```python
from build123d import *

# Parameters (mm, degrees)
F0_W        = 35
F0_H        = 20
F1_DEPTH    = 20
F2_W        = 30
F2_H        = 17.5
F3_DEPTH    = 25
F4_R        = 6
F5_DEPTH    = 5
F6_T1_DEPTH = 32.5
F7_R        = 7.5
F7_R_2      = 1.25
F8_DEPTH    = 25
F9_R        = 1.25
F10_DEPTH   = 25
F11_DEPTH   = 5
F13_DEPTH   = 5


# Not quite as in the source:
# - a fillet or chamfer that OpenCascade refuses, or shapes differently, is made with other operations: its cross-section is extruded or revolved along the edge and cut away or added


with BuildPart() as f1:
    # F0 (on Top) → F1 (new body)
    with BuildSketch(Plane.XY):
        with Locations((17.5, 10)):
            Rectangle(F0_W, F0_H)
    extrude(amount=F1_DEPTH)

    # F2 (on face) → F3 (cut)
    with BuildSketch(Plane.XY.offset(20)):
        with Locations((17.5, 11.25)):
            Rectangle(F2_W, F2_H)
    extrude(amount=-F3_DEPTH, mode=Mode.SUBTRACT)

    # F4 (on face) → F5 (cut)
    with BuildSketch(Plane(origin=(0, 0, 0), x_dir=(0, -1, 0), z_dir=(-1, 0, 0))):
        with Locations((-7.5, 10)):
            Circle(F4_R)
        Polygon((-20, 20), (-20, 10), (-10, 20), align=None)
    extrude(amount=-F5_DEPTH, mode=Mode.SUBTRACT)

    # F6: fillet of radius 2.5 on 2 edges, made by hand

    # F6_s2 → F6_t1 (cut)
    with BuildSketch(Plane.XY.offset(-6.25)):
        with BuildLine():
            ThreePointArc((0, 2.5), (0.732233047, 0.732233047), (2.5, 0))
            Line((2.5, 0), (0, 0))
            Line((0, 0), (0, 2.5))
        make_face()
        with BuildLine():
            ThreePointArc((32.5, 0), (34.267766953, 0.732233047), (35, 2.5))
            Line((35, 2.5), (35, 0))
            Line((35, 0), (32.5, 0))
        make_face()
    extrude(amount=F6_T1_DEPTH, mode=Mode.SUBTRACT)

    # F7 (on face) → F8 (cut)
    with BuildSketch(Plane.XZ):
        with Locations((17.5, 10)):
            Circle(F7_R)
        with Locations((28.5, 16)):
            Circle(F7_R_2)
        with Locations((28.5, 10)):
            Circle(F7_R_2)
        with Locations((28.5, 4)):
            Circle(F7_R_2)
    extrude(amount=-F8_DEPTH, mode=Mode.SUBTRACT)

    # F9 (on face) → F10 (cut)
    with BuildSketch(Plane.XZ):
        with Locations((6.5, 4)):
            Circle(F9_R)
        with Locations((6.5, 10)):
            Circle(F9_R)
        with Locations((6.5, 16)):
            Circle(F9_R)
    extrude(amount=-F10_DEPTH, mode=Mode.SUBTRACT)

    # F11 (add): a face of the model
    f11_faces = [f1.faces().sort_by_distance(p)[0] for p in [
        (33.75, 20, 10),
    ]]
    extrude(f11_faces, amount=F11_DEPTH)

    # F12 (on face) → F13 (cut)
    with BuildSketch(Plane.YZ.offset(35)):
        with BuildLine():
            Line((8, 7.5), (20, 7.5))
            ThreePointArc((20, 7.5), (22.5, 10), (20, 12.5))
            Line((20, 12.5), (8, 12.5))
            ThreePointArc((8, 12.5), (5.5, 10), (8, 7.5))
        make_face()
        with BuildLine():
            Line((15.75, 16), (25, 16))
            Line((25, 16), (25, 20))
            Line((25, 20), (13.75, 20))
            Line((13.75, 20), (13.75, 18))
            ThreePointArc((13.75, 18), (14.3357864376, 16.5857864376), (15.75, 16))
        make_face()
        with BuildLine():
            Line((25, 0), (25, 4))
            Line((25, 4), (15.75, 4))
            ThreePointArc((15.75, 4), (14.3357864376, 3.4142135624), (13.75, 2))
            Line((13.75, 2), (13.75, 0))
            Line((13.75, 0), (25, 0))
        make_face()
    extrude(amount=-F13_DEPTH, mode=Mode.SUBTRACT)


solid = f1.part
```
The listing builds one solid part. Answer for the finished solid, in the listing's coordinates (mm). A direction names the side the tool comes from. Coordinates: 2 decimals unless noted, no trailing zeros. Order: outer loops, then holes, each group sorted by start corner. A loop starts at its lowest first (then second) coordinate and runs counter-clockwise, first axis right, second up. Notation, with made-up numbers: M 46,-23 L 57,-23 A19 cw 57,-13 Z; hole C -34.75,-28.75 d4. An arc over 180 degrees is marked long. Answer as a JSON object with one key per item and string values. Group by question number.
1. Straight lines are drawn through the part: line 1 (Z direction, x = 28.5, y = 1.65); line 2 (X direction, y = 6, z = 18.5); line 3 (Z direction, x = 33, y = 10.75). For each, find the intervals that lie inside material, in ascending order.
2. Section D-D on x = 15 is taken. Write down the section's boundary in (y, z), then the cut area to 3 significant figures.
3. Section C-C on z = 12 is taken. Write down the section's boundary in (x, y).
4. Section A-A on y = 17 is taken. Write down the section's boundary in (x, z), then the cut area to 3 significant figures.
5. Section B-B on x = 6.5 is taken. Write down the section's boundary in (y, z).
6. Determine the mould class of faces 5 (the cylindrical face through (1.909, 1.777, 11.802)), 6 (the flat face through (14, 0, 3)), 7 (the flat face through (17, 2, 20)) for opening direction Z: released by +Z, released by -Z, zero draft, split by the parting line, or undercut.
7. A tool of negligible diameter and unlimited length cuts with its end or side. For faces 1 (the flat face through (2.5, 13, 6)), 2 (the flat face through (34, 14, 12.5)), 3 (the cylindrical face through (33.77, 14.35, 3.43)), 4 (the flat face through (0, 13, 5)), from which of +Z, -Z, +X, -X, +Y, -Y can it reach the whole face along a straight path? Write none if from no direction.
8. Flat-ended cylindrical pins translate along their axes: P1, Ø2, axis at x = 34, y = 17, coming from the +Z side; P2, Ø0.6, axis at x = 33.5, z = 19, coming from the +Y side; P3, Ø1.5, axis at x = 28.5, z = 4, coming from the -Y side; P4, Ø0.8, axis at x = 33.5, y = 21, coming from the -Z side. Find the tip coordinate at first contact, or state that the pin passes through.
Values follow:
{
 "1": {"line 1": "0 to 2.75, 5.25 to 8.75, 11.25 to 14.75, 17.25 to 20", "line 2": "0 to 2.5, 32.5 to 35", "line 3": "0 to 7.5, 12.5 to 20"},
 "2": {"outline": "M 0,0 L 2.5,0 L 2.5,2.93 L 0,2.93 Z; M 0,17.07 L 2.5,17.07 L 2.5,20 L 0,20 Z", "area": "14.6 mm2"},
 "3": {"outline": "M 0,13.16 L 2.5,13.16 L 2.5,18 L 0,18 Z; M 0.09,1.84 A2.5 ccw 2.5,0 L 10.27,0 L 10.27,2.5 L 5,2.5 L 5,1.84 Z; M 24.73,0 L 32.5,0 A2.5 ccw 35,2.5 L 35,6.5 L 32.5,6.5 L 32.5,2.5 L 24.73,2.5 Z; M 32.5,21.5 L 35,21.5 L 35,25 L 32.5,25 Z"},
 "4": {"outline": "M 0,0 L 2.5,0 L 2.5,13 L 0,13 Z; M 32.5,4 L 35,4 L 35,7.5 L 32.5,7.5 Z; M 32.5,12.5 L 35,12.5 L 35,16 L 32.5,16 Z", "area": "50.0 mm2"},
 "5": {"outline": "M 0,0 L 2.5,0 L 2.5,2.75 L 0,2.75 Z; M 0,5.25 L 2.5,5.25 L 2.5,8.75 L 0,8.75 Z; M 0,11.25 L 2.5,11.25 L 2.5,14.75 L 0,14.75 Z; M 0,17.25 L 2.5,17.25 L 2.5,20 L 0,20 Z"},
 "6": {"face 5": "undercut", "face 6": "zero draft", "face 7": "released by +Z"},
 "7": {"face 1": "+Z, -Z, +Y", "face 2": "+X", "face 3": "-Z, +X, +Y", "face 4": "+Z, -Z, -X, +Y, -Y"},
 "8": {"P1": "z = 16", "P2": "y = 13.75", "P3": "through", "P4": "z = 4"}
}
